from build123d import *

# Parameters (mm, degrees)
F1_DEPTH = 3
F2_R     = 2


with BuildPart() as f1:
    # F0 (on Top) → F1 (new body)
    with BuildSketch(Plane.XY):
        Polygon((-8.146908, 7.150882), (-18.146908, 7.150882), (-18.146908, -3.36134), (-8.146908, -12.728843), align=None)
        Polygon((61.853092, 7.150882), (-8.146908, 7.150882), (-8.146908, -12.728843), (-8.146908, -32.849118), (61.853092, -32.849118), (61.853092, -12.849118), align=None)
        Polygon((71.853092, -21.79648), (61.853092, -12.849118), (61.853092, -32.849118), (71.853092, -32.849118), align=None)
    extrude(amount=F1_DEPTH)

    # F2
    f2_edges = [f1.edges().sort_by_distance(p)[0] for p in [
        (-18.146908, 7.150882, 1.5),
        (-18.146908, -3.36134, 1.5),
        (-8.146908, -12.728843, 1.5),
        (-8.146908, -32.849118, 1.5),
        (71.853092, -32.849118, 1.5),
        (71.853092, -21.79648, 1.5),
        (61.853092, -12.849118, 1.5),
        (61.853092, 7.150882, 1.5),
    ]]
    fillet(f2_edges, radius=F2_R)


solid = f1.part
Verification items for the finished model (mm, model axes). A direction names the side the tool comes from. Give positions to 0.01 mm unless a question says otherwise; leave off trailing zeros. Loops run counter-clockwise (first coordinate to the right, second up) from the corner with the lowest first, then second, coordinate; pieces in that order, holes last.
1) Sectioned sample at C-C, the plane y = -18. Enter the section's corners in (x, z), then the cut area to 3 significant figures.
2) Thickness scan on line 1 along X through (y, z) = (-25.5, 1.9); line 2 along X through (y, z) = (5, 1.55); line 3 along Y through (x, z) = (64.5, 1.95). Record the ranges inside material, lowest first.
3) Sectioned sample at A-A, the plane z = 2. Enter the section's corners in (x, y).
4) Set-up check for faces 1 (the flat face through (-8.147, -22, 1)), 2 (the flat face through (26, -13, 3)), 3 (the flat face through (61.853, -4, 1)): record each of +Z, -Z, +X, -X, +Y, -Y from which the full face is reachable in a straight line by a thin tool's end or side.
5) Sectioned sample at B-B, the plane y = 4. Enter the section's corners in (x, z).
6) Depth check by flat-ended pin: pin 1 Ø8 at (x, y) = (26, -19) entering from -Z. Enter the tip coordinate at first touch or a pass-through.
Answers:
1. outline: (-8.15, 0) - (67.61, 0) - (67.61, 3) - (-8.15, 3) - close
1. area: 227 mm2
2. line 1: x = -8.15 to 71.85
2. line 2: x = -18.15 to 61.85
2. line 3: y = -32.85 to -15.22
3. outline: (-18.15, -2.49) arc R2 ccw to (-17.51, -3.95) - (-8.78, -12.14) arc R2 cw to (-8.15, -13.6) - (-8.15, -30.85) arc R2 ccw to (-6.15, -32.85) - (69.85, -32.85) arc R2 ccw to (71.85, -30.85) - (71.85, -22.69) arc R2 ccw to (71.19, -21.2) - (62.52, -13.45) arc R2 cw to (61.85, -11.95) - (61.85, 5.15) arc R2 ccw to (59.85, 7.15) - (-16.15, 7.15) arc R2 ccw to (-18.15, 5.15) - close
4. face 1: +Z, -Z, -X, -Y
4. face 2: +Z, +X, -X, +Y, -Y
4. face 3: +Z, -Z, +X, +Y
5. outline: (-18.15, 0) - (61.85, 0) - (61.85, 3) - (-18.15, 3) - close
6. pin 1: stops at z = 0
